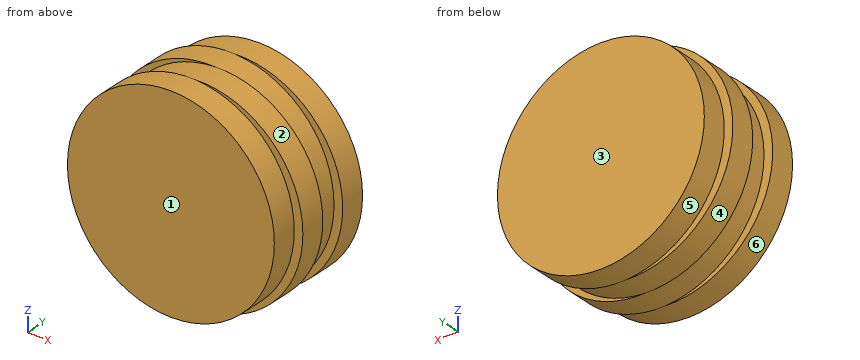
from build123d import *

# Parameters (mm, degrees)
SKETCH1_R           = 36
BOSS_EXTRUDE1_DEPTH = 9
SKETCH2_R           = 36
BOSS_EXTRUDE2_DEPTH = 9
SKETCH3_R           = 36
BOSS_EXTRUDE3_DEPTH = 9
SKETCH4_R           = 36
BOSS_EXTRUDE4_DEPTH = 9


with BuildPart() as part:
    # Sketch1 → Boss-Extrude1 (new body)
    with BuildSketch(Plane(origin=(0, 0, 0), x_dir=(1, 0, 0), z_dir=(0, 1, 0))):
        Circle(SKETCH1_R)
    extrude(amount=BOSS_EXTRUDE1_DEPTH)

    # Sketch2 → Boss-Extrude2 (add)
    with BuildSketch(Plane(origin=(0, 9, 0), x_dir=(1, 0, 0), z_dir=(0, 1, 0))):
        with Locations((3, 0)):
            Circle(SKETCH2_R)
    extrude(amount=BOSS_EXTRUDE2_DEPTH)

    # Sketch3 → Boss-Extrude3 (add)
    with BuildSketch(Plane(origin=(0, 18, 0), x_dir=(1, 0, 0), z_dir=(0, 1, 0))):
        Circle(SKETCH3_R)
    extrude(amount=BOSS_EXTRUDE3_DEPTH)

    # Sketch4 → Boss-Extrude4 (add)
    with BuildSketch(Plane(origin=(0, 27, 0), x_dir=(1, 0, 0), z_dir=(0, 1, 0))):
        with Locations((3, 0)):
            Circle(SKETCH4_R)
    extrude(amount=BOSS_EXTRUDE4_DEPTH)


solid = part.part
Build history of the part. All positions in model axes, mm. Face numbers are marked on the shaded views. A direction names the side the tool comes from. Give positions to 0.01 mm unless a question says otherwise; leave off trailing zeros. Order: outer loops, then holes, each group sorted by start corner. A loop starts at its lowest first (then second) coordinate and runs counter-clockwise, first axis right, second up. Notation, with made-up numbers: M -14.75,0.5 L 7.25,0.5 A18 cw 7.25,27.5 Z; hole C -35,-35 d8. An arc over 180 degrees is marked long. Use one line per item in the form item = value.
Q1. Which spindle directions (+Z, -Z, +X, -X, +Y, -Y) get a long thin tool onto all of the face, cutting with end or side? Do the marked faces 4, 5 and 6. Say none if no direction does.
Conclusion:
face_4 = none
face_5 = +Y
face_6 = -Y
Q2. Slice it at A-A, the plane z = 0. Write the cut outline in (x, y).
Conclusion:
outline = M -36,0 L 36,0 L 36,9 L 39,9 L 39,18 L 36,18 L 36,27 L 39,27 L 39,36 L -33,36 L -33,27 L -36,27 L -36,18 L -33,18 L -33,9 L -36,9 Z
Q3. Slice it at B-B, the plane x = -27. Write the cut outline in (y, z).
Conclusion:
outline = M 0,-23.81 L 9,-23.81 L 9,-19.9 L 18,-19.9 L 18,-23.81 L 27,-23.81 L 27,-19.9 L 36,-19.9 L 36,19.9 L 27,19.9 L 27,23.81 L 18,23.81 L 18,19.9 L 9,19.9 L 9,23.81 L 0,23.81 Z
Q4. Wall check: probe 1 along Y at (x, z) = (33, -18.5); probe 2 along X at (y, z) = (6, 0.5); probe 3 along X at (y, z) = (32, 1). Give the ranges that are in metal, low to high.
Conclusion:
probe_1 = 9 to 18, 27 to 36
probe_2 = -36 to 36
probe_3 = -32.99 to 38.99
Q5. Pin check, flat tips, straight feed: P1, Ø3, axis at x = -0.5, y = 15, coming from the +Z side; P2, Ø2, axis at x = -5, y = 6, coming from the +Z side; P3, Ø10, axis at x = -22, y = 12, coming from the -Z side. Stop position of each tip, or through.
Conclusion:
P1 = 35.94
P2 = 35.78
P3 = -31.18
Q6. Pull direction Y, two halves, no side cores. Call the marked faces 1, 2 and 3: released by +Y, released by -Y, zero draft, split by the parting line, or undercut.
Conclusion:
face_1 = released by -Y
face_2 = undercut
face_3 = released by +Y
Q7. Slice it at C-C, the plane y = 7.5. Write the cut outline in (x, z), and give its area (3 significant figures).
Conclusion:
outline = C 0,0 d72
area = 4,070 mm2
